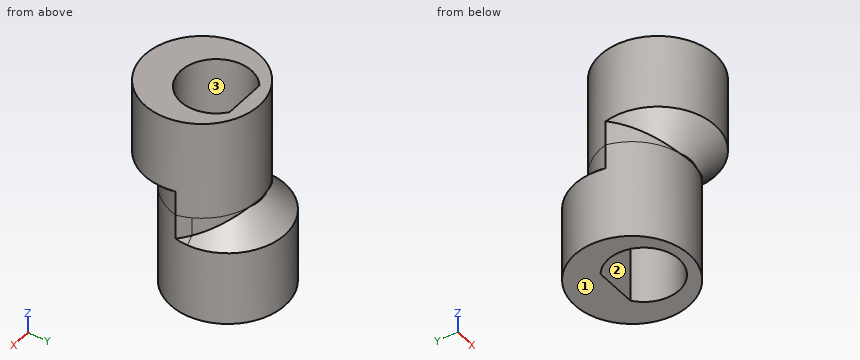
```python
from build123d import *

# Parameters (mm, degrees)
ESQUISSE1_R             = 4.05
BOSS_EXTRU_1_DEPTH      = 7
ESQUISSE2_R             = 4.05
BOSS_EXTRU_2_DEPTH      = 7
ENL_V_MAT_EXTRU_1_DEPTH = 16.424169346
CHANFREIN2_SIZE         = 1.75
CHANFREIN4_SIZE         = 1.75


with BuildPart() as part:
    # Esquisse1 → Boss.-Extru.1 (new body)
    with BuildSketch(Plane.XY):
        with Locations((0, 0.822072072)):
            Circle(ESQUISSE1_R)
    extrude(amount=BOSS_EXTRU_1_DEPTH)

    # Esquisse2 → Boss.-Extru.2 (add)
    with BuildSketch(Plane.XY.offset(7)):
        with Locations(Location((0, -1, 0), (0, 0, 167.000228446))):
            Circle(ESQUISSE2_R)
    extrude(amount=BOSS_EXTRU_2_DEPTH)

    # Esquisse3 → Enlèv. mat.-Extru.1 (cut, through all)
    with BuildSketch(Plane.XY.offset(14)):
        with BuildLine():
            Line((-1.5, 2), (1.5, 2))
            ThreePointArc((1.5, 2), (0, -2.5), (-1.5, 2))
        make_face()
    extrude(amount=-ENL_V_MAT_EXTRU_1_DEPTH, mode=Mode.SUBTRACT)

    # Chanfrein2
    # the kernel refuses this chamfer: 1.75 mm, written as the material it takes off along each edge
    with BuildSketch(Plane(origin=(0, 0.822072072, 7), x_dir=(1, 0, 0), z_dir=(0, -1, 0))) as chanfrein2_piece_1_section:
        Polygon((4.05, -CHANFREIN2_SIZE), (4.05 - CHANFREIN2_SIZE, 0), (4.05, 0), align=None)
    chanfrein2_piece_1 = revolve(axis=Axis((0, 0.822072072, 7), (0, 0, 1)), revolution_arc=256.785781501, mode=Mode.PRIVATE)
    chanfrein2_piece_1 = chanfrein2_piece_1 - Plane(origin=(0, -1, 6.142651894), x_dir=(-0.9743709616876816, 0.22494716939722223, 0), z_dir=(0, 0, -1)) * Cylinder(4.05, 17, mode=Mode.PRIVATE)
    add(chanfrein2_piece_1, mode=Mode.SUBTRACT)
    with BuildSketch(Plane(origin=(0, 0.822072072, 7), x_dir=(0.23058336065371998, -0.9730525750387985, 0), z_dir=(-0.9730525750387985, -0.23058336065371998, 0))) as chanfrein2_piece_2_section:
        Polygon((4.05, -CHANFREIN2_SIZE), (4.05 - CHANFREIN2_SIZE, 0), (4.05, 0), align=None)
    chanfrein2_piece_2 = revolve(axis=Axis((0, 0.822072072, 7), (0, 0, 1)), revolution_arc=76.66858095, mode=Mode.PRIVATE)
    chanfrein2_piece_2 = chanfrein2_piece_2 - Plane(origin=(0, -1, 6.19314211), x_dir=(-0.9743709616876816, 0.22494716939722223, 0), z_dir=(0, 0, -1)) * Cylinder(4.05, 17, mode=Mode.PRIVATE)
    add(chanfrein2_piece_2, mode=Mode.SUBTRACT)

    # Chanfrein4
    # the kernel refuses this chamfer: 1.75 mm, written as the material it takes off along each edge
    with BuildSketch(Plane(origin=(0, -1, 7), x_dir=(-0.22831348546058428, 0.9735876706064225, 0), z_dir=(0.9735876706064225, 0.22831348546058428, 0))) as chanfrein4_piece_1_section:
        Polygon((4.05 - CHANFREIN4_SIZE, 0), (4.05, CHANFREIN4_SIZE), (4.05, 0), align=None)
    chanfrein4_piece_1 = revolve(axis=Axis((0, -1, 7), (0, 0, 1)), revolution_arc=333.604400204, mode=Mode.PRIVATE)
    chanfrein4_piece_1 = chanfrein4_piece_1 - Plane(origin=(0, 0.822072072, 7.857230716), x_dir=(1, 0, 0), z_dir=(0, 0, -1)) * Cylinder(4.05, 17, mode=Mode.PRIVATE)
    add(chanfrein4_piece_1, mode=Mode.SUBTRACT)


solid = part.part
```
Can you work these out from the model? Positions are in its coordinate system, mm. Face numbers are marked on the shaded views. Coordinates: 2 decimals unless noted, no trailing zeros. Order: outer loops, then holes, each group sorted by start corner. A loop starts at its lowest first (then second) coordinate and runs counter-clockwise, first axis right, second up.
1. If we section it at B-B (z = 2.5): Please give me the cut outline in (x, y), then the cut area to 3 significant figures.
2. I'm going to push flat-ended pins straight in: pin 1 (1 mm diameter, centred on y = 3, z = 11, fed in from -X); pin 2 (2 mm diameter, centred on y = -3.5, z = 11.5, fed in from -X); pin 3 (2.5 mm diameter, centred on x = -0.5, z = 4, fed in from -Y). Where does each tip first touch, or does it pass through?
3. If we section it at C-C (y = -1): Please give me the cut outline in (x, z).
4. If we section it at A-A (x = 0): Please give me the cut outline in (y, z), then the cut area to 3 significant figures.
5. If we section it at D-D (z = 6): Please give me the cut outline in (x, y).
6. I need wall thicknesses on line 1 (Y direction, x = 0, z = 3.5); line 2 (Y direction, x = 0, z = 6.5); line 3 (X direction, y = 0, z = 8.5). Which ranges of each line are inside material? Lowest first, please.
7. Thinking about a two-plate mould opening in Y: for the marked faces 1, 2 and 3, which applies, +Y half, -Y half, draft (parallel to the pull), parting line (faces both ways), or undercut?
Entries:
1. outline: circle Ø8.1 at (0, 0.82); hole (-1.5, 2) arc R2.5 ccw (long way) to (1.5, 2) - close
1. area: 32.9 mm2
2. pin 1: stops at x = -2.04
2. pin 2: stops at x = -3.76
2. pin 3: stops at y = -3.23
3. outline: (-4.05, 8.75) - (-3.62, 8.32) - (-3.62, 0) - (-2.29, 0) - (-2.29, 14) - (-4.05, 14) - close; (2.29, 0) - (3.62, 0) - (3.62, 8.32) - (4.05, 8.75) - (4.05, 14) - (2.29, 14) - close
4. outline: (-5.05, 8.75) - (-3.3, 7) - (-3.23, 7) - (-3.23, 0) - (-2.5, 0) - (-2.5, 14) - (-5.05, 14) - close; (2, 0) - (4.87, 0) - (4.87, 5.25) - (3.12, 7) - (3.05, 7) - (3.05, 14) - (2, 14) - close
4. area: 47.3 mm2
5. outline: (-3.95, -0.09) arc R4.05 ccw to (3.95, -0.09) arc R4.05 ccw to (3.24, 1.42) arc R3.3 ccw to (-3.24, 1.42) arc R4.05 ccw to start; hole (-1.5, 2) arc R2.5 ccw (long way) to (1.5, 2) - close
6. line 1: y = -3.23 to -2.5, 2 to 4.87
6. line 2: y = -3.23 to -2.5, 2 to 3.62
6. line 3: x = -3.92 to -2.5, 2.5 to 3.92
7. face 1: draft
7. face 2: undercut
7. face 3: undercut
